Geometry: final body of the model. Coordinates: model frame, mm. A direction names the side the tool comes from. Coordinates: 2 decimals unless noted, no trailing zeros. Loops run counter-clockwise (first coordinate to the right, second up) from the corner with the lowest first, then second, coordinate; pieces in that order, holes last. Notation, with made-up numbers: (39.25, -11) - (49.25, -11) arc R23 ccw to (49.25, 25) - close; hole circle Ø2 at (26.5, 38). An arc over 180 degrees is marked (long way). Return JSON: item names as keys, results as strings.
Autodesk Inventor part; units mm, degrees
ref_plane "Work Plane1" through (0, 17, 65) normal (0, 1, 0) x (-1, 0, 0)
ref_plane "YZ Plane" through (0, 0, 0) normal (1, 0, 0) x (0, 1, 0)
ref_plane "XZ Plane" through (0, 0, 0) normal (0, 1, 0) x (-1, 0, 0)
sketch "Sketch1" plane through (0, 0, 0) normal (0, 0, 1) x (1, 0, 0)
  circle A0 centre (0, 0) radius 18.5
  arc A1 (-8.9075, 7.6329) -> (8.9075, 7.6329) centre (0, 7) ccw
  spline S0 degree 3 poles (8.9075, 7.6329) (8.9044, 7.6769) (8.9082, 7.7215) (8.9387, 7.8037) (8.9677, 7.8415) (9.0503, 7.8747) (9.0975, 7.8677) (9.1766, 7.8302) (9.2105, 7.8009) (9.2388, 7.7672) knots 0 0 0 0 0.25 0.25 0.5 0.5 0.75 0.75 1 1 1 1
  arc A2 (-9.2388, 7.7672) -> (9.2388, 7.7672) centre (0, 0) ccw
  spline S1 degree 3 poles (-9.2388, 7.7672) (-9.2105, 7.801) (-9.1766, 7.8302) (-9.0974, 7.8677) (-9.0502, 7.8747) (-8.9678, 7.8415) (-8.9387, 7.8036) (-8.9082, 7.7215) (-8.9044, 7.6769) (-8.9075, 7.6329) knots 0 0 0 0 0.25 0.25 0.5 0.5 0.75 0.75 1 1 1 1
  circle A3 centre (7.75, -13.4234) radius 1.6
  circle A4 centre (-7.75, -13.4234) radius 1.6
  circle A5 centre (-15.5, 0) radius 1.6
  circle A6 centre (-7.75, 13.4234) radius 1.6
  circle A7 centre (7.75, 13.4234) radius 1.6
  circle A8 centre (15.5, 0) radius 1.6
  circle A9 centre (13.4234, 7.75) radius 2.1
  circle A10 centre (-13.4234, 7.75) radius 2.1
  circle A11 centre (0, -15.5) radius 2.1
  circle A12 centre (0, 7) radius 6.25
  line L0 (20, -25) -> (-20, -25)
  line L1 (-20, -25) -> (-20, 25)
  line L2 (-20, 25) -> (20, 25)
  line L3 (20, 25) -> (20, -25)
  line L4 (20, -25) -> (-20, 25) construction
  line L5 (-20, -25) -> (20, 25) construction
  dimension "d0" = 40
  dimension "d1" = 50
extrude "Extrusion1" add sketch "Sketch1" along normal blind 2 contours A0 | A1 S0 A2 S1 | A9 | A10 | A11 | L0 L1 L2 L3
sketch "Sketch2" plane through (0, 0, 2) normal (0, 0, 1) x (1, 0, 0)
  line L0 (-20, -25) -> (20, -25)
  line L1 (20, -25) -> (-20, -25)
  line L2 (-20, -25) -> (-20, -27)
  line L3 (-20, -27) -> (20, -27)
  line L4 (20, -27) -> (20, -25)
  line L5 (20, 25) -> (-20, 25)
  line L6 (20, 25) -> (-20, 25)
  line L7 (-20, 25) -> (-20, 27)
  line L8 (-20, 27) -> (20, 27)
  line L9 (20, 27) -> (20, 25)
  point P0 (0, 0)
  dimension "d4" = 2
  dimension "d19" = 2
extrude "Extrusion2" add sketch "Sketch2" against normal blind 70
sketch "Sketch5" plane through (0, 0, -68) normal (0, 0, -1) x (-1, 0, 0)
  line L0 (-20, -27) -> (20, -27)
  line L1 (20, -27) -> (20, 27)
  line L2 (20, 27) -> (-20, 27)
  line L3 (-20, 27) -> (-20, -27)
  circle A0 centre (0, 7) radius 6 construction
  circle A1 centre (0, 7) radius 3 construction
  circle A2 centre (0, 17) radius 1.5
  circle A3 centre (-8.6603, 2) radius 1.5
  circle A4 centre (8.6603, 2) radius 1.5
  point P0 (0, 0)
  dimension "d20" = 10
  dimension "d21" = 3
  dimension "d24" = 360
extrude "Extrusion4" add sketch "Sketch5" along normal blind 2
sketch "Sketch6" plane through (0, 0, 2) normal (0, 0, 1) x (1, 0, 0)
  line L0 (20, -27) -> (20, 27)
  line L1 (-20, -27) -> (20, -27)
  line L2 (20, -27) -> (20, -20)
  line L3 (20, -20) -> (-20, -20)
  line L4 (-20, -20) -> (-20, -27)
  circle A0 centre (0, 0) radius 18.5
  point P0 (0, 0)
  dimension "d28" = 7
extrude "Extrusion5" cut sketch "Sketch6" against normal up to surface (72 mm away) contours L1 L4 L3 L0
sketch "Sketch7" plane through (0, 0, 2) normal (0, 0, 1) x (1, 0, 0)
  line L0 (-20, 27) -> (-20, -20)
  line L1 (20, -20) -> (20, 27)
  line L2 (-20, -20) -> (20, -20)
  line L3 (20, -20) -> (20, -22)
  line L4 (20, -22) -> (-20, -22)
  line L5 (-20, -22) -> (-20, -20)
  point P0 (0, 0)
  dimension "d31" = 2
extrude "Extrusion6" add sketch "Sketch7" against normal up to surface (72 mm away)
sketch "Sketch8" plane through (0, 0, 2) normal (0, 0, 1) x (1, 0, 0)
  circle A0 centre (0, 22) radius 2.5
  circle A1 centre (0, -8) radius 2.5
  point P0 (0, 0)
  dimension "d34" = 22
  dimension "d35" = 5
  dimension "d36" = 8
extrude "Extrusion7" add sketch "Sketch8" along normal blind 46
sketch "Sketch11" plane through (0, 22, 48) normal (0, 0, 1) x (1, 0, 0)
  circle A0 centre (0, -15) radius 8 construction
  circle A1 centre (0, -15) radius 20
  circle A2 centre (0, -15) radius 11
  point P0 (0, -22)
  dimension "d44" = 40
  dimension "d45" = 22
extrude "Extrusion9" add sketch "Sketch11" against normal blind 5
sketch "Sketch14" plane through (0, 7, 48) normal (0, 0, 1) x (1, 0, 0)
  circle A0 centre (-15, 0) radius 2
  circle A1 centre (0, 0) radius 6.282 construction
  circle A2 centre (15, 0) radius 2
  point P0 (0, -7)
  dimension "d60" = 15
  dimension "d61" = 4
  dimension "d64" = 360
extrude "Extrusion12" add sketch "Sketch14" along normal blind 15
sketch "Sketch15" plane through (-15, 7, 63) normal (0, 0, 1) x (1, 0, 0)
  circle A0 centre (15, 0) radius 4 construction
  circle A1 centre (15, 0) radius 11 construction
  circle A2 centre (15, 0) radius 20
  circle A3 centre (15, 0) radius 20
  circle A4 centre (15, 0) radius 5
  point P0 (15, -7)
  dimension "d68" = 40
  dimension "d69" = 10
extrude "Extrusion13" add sketch "Sketch15" along normal blind 2
sketch "Sketch16" plane through (0, 7, 65) normal (0, 0, 1) x (1, 0, 0)
  circle A0 centre (0, 0) radius 5 construction
  circle A1 centre (0, 0) radius 7.5
  circle A2 centre (0, 0) radius 11 construction
  circle A3 centre (0, 0) radius 10
  point P0 (0, -7)
  dimension "d72" = 15
  dimension "d73" = 20
extrude "Extrusion14" add sketch "Sketch16" along normal blind 137.5
ref_plane "Work Plane1" through (0, 17, 65) normal (0, 1, 0) x (-1, 0, 0)
sketch "Sketch17" plane through (0, 17, 65) normal (0, 1, 0) x (-1, 0, 0)
  line L0 (2, 133.5) -> (-2, 133.5)
  line L1 (-2, 133.5) -> (-2, 4)
  line L2 (-2, 4) -> (2, 4)
  line L3 (2, 4) -> (2, 133.5)
  line L4 (-10, 0) -> (-10, 137.5)
  line L5 (10, 0) -> (10, 137.5)
  line L6 (10, 137.5) -> (-10, 137.5)
  line L7 (-10, 0) -> (10, 0)
  point P0 (0, -65)
  dimension "d76" = 4
  dimension "d77" = 4
  dimension "d78" = 8
  dimension "d79" = 8
extrude "Extrusion15" cut sketch "Sketch17" against normal up to surface contours L3 L2 L1 L0
sketch "Sketch18" plane through (0, 0, -70) normal (0, 0, -1) x (-1, 0, 0)
  circle A0 centre (0, 7) radius 6 construction
  circle A1 centre (0, 7) radius 14
  circle A2 centre (0, 17) radius 1.5
  circle A3 centre (-8.6603, 2) radius 1.5
  circle A4 centre (8.6603, 2) radius 1.5
  point P0 (0, 0)
  dimension "d82" = 28
extrude "Extrusion16" add sketch "Sketch18" along normal blind 2.5
sketch "Sketch19" plane through (0, 7, -72.5) normal (0, 0, -1) x (-1, 0, 0)
  circle A0 centre (0, 0) radius 14 construction
  circle A1 centre (0, 0) radius 3.3
  point P0 (0, -7)
  point P1 (-1.4736, 13.9222)
  point P2 (1.4736, 13.9222)
  dimension "d85" = 6.6
extrude "Extrusion17" add sketch "Sketch19" along normal blind 10
properties part number "motor bracket"
Item 1: First-contact query: pin 1 Ø4 at (x, y) = (-15.5, 0) entering from -Z; pin 2 Ø1.3 at (y, z) = (15.5, 144) entering from +X; pin 3 Ø20 at (x, y) = (-8, -1) entering from +Z; pin 4 Ø3 at (x, y) = (-7.75, 13.42) entering from -Z. Flat tips, straight axial feed; report the tip coordinate or a pass-through.
Worked out:
{"pin 1": "z = -70", "pin 2": "x = 6.19", "pin 3": "z = 202.5", "pin 4": "z = -72.5"}
Item 2: Reachability of faces 5 (the face through (0, -20, -34)), 6 (the face through (5.96, 5.12, 0.99)), 7 (the face through (-2.6, 26.83, 45.54)) from +Z, -Z, +X, -X, +Y, -Y: full face, straight path, thin tool, end or side. Return the list, or none.
Worked out:
{"face 5": "+X, -X", "face 6": "none", "face 7": "+Z"}
Item 3: Mould query, pull axis Y, two halves, no side actions, for faces 1 (the face through (0, -22, -33)), 2 (the face through (-0.33, 19.52, 22.21)), 3 (the face through (4.614, 15.872, 132.788)), 4 (the face through (0, 7, -82.5)). Classes: +Y half, -Y half, draft (parallel to the pull), parting line (faces both ways), or undercut.
Worked out:
{"face 1": "-Y half", "face 2": "undercut", "face 3": "parting line", "face 4": "draft"}
Item 4: Section query A-A, the plane z = -35. Return loops of the section in (x, y), and give its area (3 significant figures).
Worked out:
{"outline": "(-20, -22) - (20, -22) - (20, -20) - (-20, -20) - close; (-20, 25) - (20, 25) - (20, 27) - (-20, 27) - close", "area": "160 mm^2"}
Item 5: Section query B-B, the plane z = 30.5. Return loops of the section in (x, y), and give its area (3 significant figures).
Worked out:
{"outline": "circle Ø5 at (0, -8); circle Ø5 at (0, 22)", "area": "39.3 mm^2"}
Item 6: Ray query, probe 1 along Z at (x, y) = (16.5, 6); probe 2 along Z at (x, y) = (18, 6); probe 3 along Z at (x, y) = (-1.5, 17.5). Return the intervals inside material, ascending. Write a range as from..to.
Worked out:
{"probe 1": "-70..-68, 0..2, 43..65", "probe 2": "-70..-68, 0..2, 43..48, 63..65", "probe 3": "-72.5..-68, 0..2, 63..65"}
Item 7: Section query C-C, the plane z = 115.5. Return loops of the section in (x, y), and give its area (3 significant figures).
Worked out:
{"outline": "(-2, 14.23) - (-2, 16.8) arc R10 ccw (long way) to (2, 16.8) - (2, 14.23) arc R7.5 cw (long way) to start", "area": "127 mm^2"}
